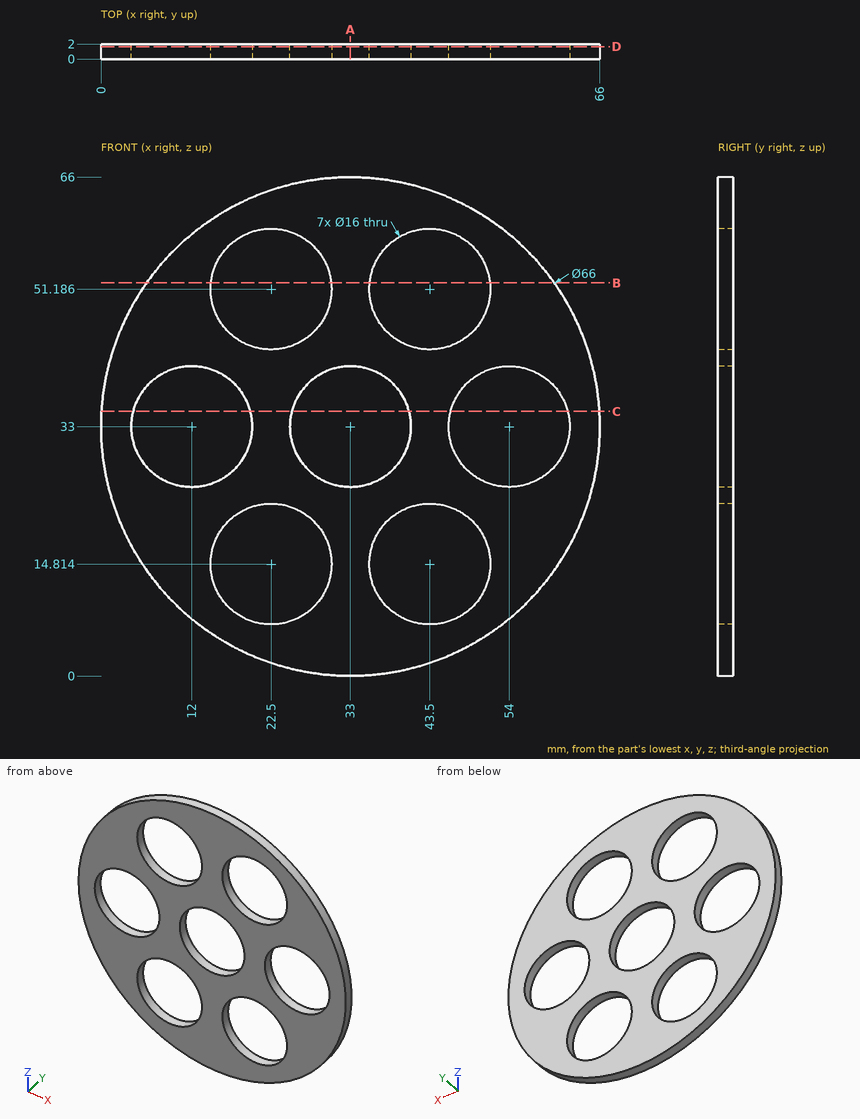
The figure shows three views and two pictorial views of one solid part (mm, origin at its lowest corner). Answer the questions. Round coordinates to 2 decimals unless told otherwise and drop trailing zeros. Order: outer loops, then holes, each group sorted by start corner. A loop starts at its lowest first (then second) coordinate and runs counter-clockwise, first axis right, second up. Notation, with made-up numbers: M 9,60 L 48,60 A18 ccw 48,91 Z; hole C 8,86.25 d4. An arc over 180 degrees is marked long. Answer in a Markdown table with one row per item. Add a question column.
1) The part is cut by section B-B on z = 52. Determine the outline of the cut face in (x, y).
2) Flat-ended cylindrical pins translate along their axes: pin 1 Ø1 at (x, y) = (49.5, 0.5) entering from -Z; pin 2 Ø1 at (y, z) = (1.5, 10.5) entering from +X (1 decimal); pin 3 Ø1 at (y, z) = (1, 25.5) entering from -X. Find the tip coordinate at first contact, or state that the pin passes through.
3) Consider line 1 along X through (y, z) = (0.35, 20.5) (1 decimal); line 2 along Z through (x, y) = (33, 0.1); line 3 along X through (y, z) = (0.85, 35) (1 decimal). Determine where each line is inside the solid, lowest interval first. Write a range as from..to.
4) The part is cut by section C-C on z = 35. Determine the outline of the cut face in (x, y) (1 decimal).
5) The part is cut by section A-A on x = 33. Determine the outline of the cut face in (y, z), plus the area to 3 significant figures.
6) The part is cut by section D-D on y = 1.65. Determine the outline of the cut face in (x, z).
Findings below:
| question | item | result |
|---|---|---|
| 1 | outline | M 6.02,0 L 14.54,0 L 14.54,2 L 6.02,2 Z; M 30.46,0 L 35.54,0 L 35.54,2 L 30.46,2 Z; M 51.46,0 L 59.98,0 L 59.98,2 L 51.46,2 Z |
| 2 | pin 1 | stops at z = 4.14 |
| 2 | pin 2 | stops at x = 57.6 |
| 2 | pin 3 | stops at x = 0.75 |
| 3 | line 1 | x = 2.5..16.9, 28.1..37.9, 49.1..63.5 |
| 3 | line 2 | z = 0..25, 41..66 |
| 3 | line 3 | x = 0.1..4.3, 19.7..25.3, 40.7..46.3, 61.7..65.9 |
| 4 | outline | M 0.1,0 L 4.3,0 L 4.3,2 L 0.1,2 Z; M 19.7,0 L 25.3,0 L 25.3,2 L 19.7,2 Z; M 40.7,0 L 46.3,0 L 46.3,2 L 40.7,2 Z; M 61.7,0 L 65.9,0 L 65.9,2 L 61.7,2 Z |
| 5 | outline | M 0,0 L 2,0 L 2,25 L 0,25 Z; M 0,41 L 2,41 L 2,66 L 0,66 Z |
| 5 | area | 100 mm² |
| 6 | outline | C 33,33 d66; hole C 12,33 d16; hole C 22.5,14.81 d16; hole C 22.5,51.19 d16; hole C 33,33 d16; hole C 43.5,14.81 d16; hole C 43.5,51.19 d16; hole C 54,33 d16 |
